from build123d import *

# Parameters (mm, degrees)
SKETCH1_R           = 2.5
BOSS_EXTRUDE1_DEPTH = 7.5
SKETCH2_R           = 3.75
BOSS_EXTRUDE2_DEPTH = 10
SKETCH3_W           = 2
SKETCH3_H           = 1
BOSS_EXTRUDE3_DEPTH = 7.5
SKETCH4_R           = 0.5
CUT_EXTRUDE1_DEPTH  = 1


with BuildPart() as part:
    # Sketch1 → Boss-Extrude1 (new body)
    with BuildSketch(Plane(origin=(0, 0, 0), x_dir=(1, 0, 0), z_dir=(0, 1, 0))):
        Polygon((-43.152827627, -30.672089533), (-35.652827627, -30.672089533), (-31.902827627, -25.672089533), (-31.902827627, -23.172089533), (-46.902827627, -23.172089533), (-46.902827627, -25.672089533), align=None)
        with Locations(Location((-39.402827627, -26.922089533, 0), (0, 0, 270))):
            Circle(SKETCH1_R, mode=Mode.SUBTRACT)
    extrude(amount=BOSS_EXTRUDE1_DEPTH)

    # Sketch2 → Boss-Extrude2 (add)
    with BuildSketch(Plane(origin=(0, 0, 23.172089533), x_dir=(-1, 0, 0), z_dir=(0, 0, -1))):
        with Locations(Location((39.402827627, 3.75, 0), (0, 0, 270))):
            Circle(SKETCH2_R)
    extrude(amount=BOSS_EXTRUDE2_DEPTH)

    # Sketch3 → Boss-Extrude3 (add)
    with BuildSketch(Plane(origin=(0, 0, 23.172089533), x_dir=(-1, 0, 0), z_dir=(0, 0, -1))):
        with Locations((45.902827627, 7)):
            Rectangle(SKETCH3_W, SKETCH3_H)
    extrude(amount=-BOSS_EXTRUDE3_DEPTH)

    # Sketch4 → Cut-Extrude1 (cut)
    with BuildSketch(Plane(origin=(0, 7.5, 0), x_dir=(1, 0, 0), z_dir=(0, 1, 0))):
        with Locations(Location((-45.902827627, -29.672089533, 0), (0, 0, 270))):
            Circle(SKETCH4_R)
    extrude(amount=-CUT_EXTRUDE1_DEPTH, mode=Mode.SUBTRACT)


solid = part.part
Source: CAD feature listing. Evaluate the final solid. Frame: model axes, mm. A direction names the side the tool comes from. Give positions to 0.01 mm unless a question says otherwise; leave off trailing zeros. Write each loop counter-clockwise with the first axis right and the second up, starting at its lowest first coordinate (ties: lowest second). Pieces come first, ordered by that corner, then holes. Notation, with made-up numbers: (-33, -13.5) -> (10, -13.5) arc R20 ccw to (10, 8.5) -> close; hole circle Ø9 at (82, 27). An arc over 180 degrees is marked (long way). Write item = value, one per line.
Q1. Line query: line 1 (Z direction, x = -40, y = 6); line 2 (Z direction, x = -40.75, y = 4.5); line 3 (X direction, y = 3.75, z = 15.75). Output: solid intervals per line, ascending. Write a range as from..to.
Here are the results:
line_1 = 13.17..24.49, 29.35..30.67
line_2 = 13.17..24.82, 29.03..30.67
line_3 = -43.15..-35.65
Q2. Reachability of faces 5 (the face through (-46, 6.5, 29)), 6 (the face through (-44.903, 7, 29)), 7 (the face through (-39, 4, 13.172)) from +Z, -Z, +X, -X, +Y, -Y: full face, straight path, thin tool, end or side. Return the list, or none.
Here are the results:
face_5 = +Z, -X, -Y
face_6 = +Z, +Y, -Y
face_7 = -Z, +X, -X, +Y, -Y
Q3. Cut plane A-A on y = 3.75. Return loops of the section in (x, z), then the cut area to 3 significant figures.
Here are the results:
outline = (-46.9, 23.17) -> (-43.15, 23.17) -> (-43.15, 13.17) -> (-35.65, 13.17) -> (-35.65, 23.17) -> (-31.9, 23.17) -> (-31.9, 25.67) -> (-35.65, 30.67) -> (-43.15, 30.67) -> (-46.9, 25.67) -> close; hole circle Ø5 at (-39.4, 26.92)
area = 149 mm²
Q4. Cut plane B-B on x = -37.5. Return loops of the section in (y, z), then the cut area to 3 significant figures.
Here are the results:
outline = (0, 23.17) -> (0.52, 23.17) -> (0.52, 13.17) -> (6.98, 13.17) -> (6.98, 23.17) -> (7.5, 23.17) -> (7.5, 25.3) -> (0, 25.3) -> close; (0, 28.54) -> (7.5, 28.54) -> (7.5, 30.67) -> (0, 30.67) -> close
area = 96.6 mm²
Q5. First-contact query: pin 1 (5 mm diameter, centred on x = -33.5, z = 16, fed in from -Y); pin 2 (4 mm diameter, centred on x = -36, z = 17.5, fed in from -Y); pin 3 (4 mm diameter, centred on y = 5.5, z = 18, fed in from +X). Flat tips, straight axial feed; report the tip coordinate or a pass-through.
Here are the results:
pin_1 = 2.17
pin_2 = 0.27
pin_3 = -35.65
Q6. Mould query, pull axis Z, two halves, no side actions, for faces 1 (the face through (-46.35, 7.01, 29.9)), 2 (the face through (-36.076, 2.02, 18.242)), 3 (the face through (-46, 7, 30.672)), 4 (the face through (-34, 4, 23.172)). Classes: +Z half, -Z half, draft (parallel to the pull), parting line (faces both ways), or undercut.
Here are the results:
face_1 = undercut
face_2 = draft
face_3 = +Z half
face_4 = -Z half
Q7. Cut plane C-C on z = 28. Return loops of the section in (x, y).
Here are the results:
outline = (-46.9, 6.5) -> (-45.16, 6.5) -> (-45.16, 0) -> (-41.66, 0) -> (-41.66, 7.5) -> (-46.9, 7.5) -> close; (-37.15, 0) -> (-33.65, 0) -> (-33.65, 7.5) -> (-37.15, 7.5) -> close
Q8. Cut plane D-D on y = 2. Return loops of the section in (x, z), then the cut area to 3 significant figures.
Here are the results:
outline = (-46.9, 23.17) -> (-42.72, 23.17) -> (-42.72, 13.17) -> (-36.09, 13.17) -> (-36.09, 23.17) -> (-31.9, 23.17) -> (-31.9, 25.67) -> (-35.65, 30.67) -> (-43.15, 30.67) -> (-46.9, 25.67) -> close; hole circle Ø5 at (-39.4, 26.92)
area = 140 mm²
